The model under review builds one solid part; all positions refer to its coordinate system, in mm. Face numbers are marked on the shaded views. A direction names the side the tool comes from. Round coordinates to 2 decimals unless told otherwise and drop trailing zeros. Loops run counter-clockwise (first coordinate to the right, second up) from the corner with the lowest first, then second, coordinate; pieces in that order, holes last. Notation, with made-up numbers: M -20,46 L 24,46 A9 ccw 24,53 Z; hole C 0,-20 d9. An arc over 180 degrees is marked long. Return JSON: item names as keys, results as strings. Group by question number.
Q1. Consider section B-B (x = -20.5). State the section outline as (y, z) points.
Q2. Consider section A-A (x = 12.7). Count the separate pieces of the cut face and the enclosed holes in it, and give its area (3 significant figures).
Q3. For the marked faces 4, 5, 6, 7 and 8, list the 3-axis set-ups (+Z, -Z, +X, -X, +Y, -Y) from which the entire face can be reached by the end or side of a thin tool; tool diameter is ignored.
Q4. To check wall thickness, follow line 1 along X through (y, z) = (12.7, 4.9); line 2 along Z through (x, y) = (-18.5, 32.5); line 3 along X through (y, z) = (32.5, -5.25). State the ranges of each line that lie inside material, in increasing order.
Q5. Draft analysis for pull direction X (two halves, no side actions). For the marked faces 1, 2 and 3, state which applies: pulls with the +X half, pulls with the -X half, needs draft (parallel to the pull), parting line crosses it, or undercut.
Q6. Clearance check with flat-ended pins moving along their axes: pin 1 Ø6 at (x, z) = (11, 4.5) entering from +Y; pin 2 Ø3.5 at (y, z) = (33.5, -2) entering from +X; pin 3 Ø3.5 at (y, z) = (16, 0) entering from -X; pin 4 Ø6 at (x, z) = (18, -3) entering from +Y. State where each tip first meets the part, or that it passes through.
from build123d import *

# Parameters (mm, degrees)
SKETCH1_W                = 38.1
SKETCH1_H                = 12.7
SKETCH1_R                = 4.05
BOSS_EXTRUDE1_DEPTH      = 25.4
SKETCH5_R                = 1.7526
CUT_EXTRUDE2_DEPTH       = 35.195796525
SKETCH6_W                = 49.584
SKETCH6_H                = 12.7
BOSS_EXTRUDE4_DEPTH      = 19.05
CUT_EXTRUDE3_DEPTH       = 67.893183937
CUT_EXTRUDE4_DEPTH       = 67.893183937
CUT_EXTRUDE5_DEPTH       = 53.194652565
CHAMFER1_SIZE            = 0.6
SKETCH10_W               = 12.7
SKETCH10_H               = 25.4
CUT_EXTRUDE6_DEPTH       = 53.194652565
CHAMFER2_SIZE            = 0.6
CHAMFER3_SIZE            = 0.3
BOSS_EXTRUDE5_DEPTH      = 1.5875
BOSS_EXTRUDE5_DEPTH_BACK = 1.5875
SKETCH14_R               = 4.7625
BOSS_EXTRUDE6_DEPTH      = 2.54
SKETCH15_R               = 1.7526
CUT_EXTRUDE7_DEPTH       = 53.870117777
CHAMFER4_SIZE            = 0.4
SKETCH18_R               = 4.1
BOSS_EXTRUDE7_DEPTH      = 6.35


with BuildPart() as part:
    # Sketch1 → Boss-Extrude1 (new body)
    with BuildSketch(Plane(origin=(0, 0, 0), x_dir=(1, 0, 0), z_dir=(0, 1, 0))):
        Rectangle(SKETCH1_W, SKETCH1_H)
        with Locations(Location((12.7, 0, 0), (0, 0, 270))):
            Circle(SKETCH1_R, mode=Mode.SUBTRACT)
        with Locations(Location((-12.7, 0, 0), (0, 0, 90))):
            Circle(SKETCH1_R, mode=Mode.SUBTRACT)
    extrude(amount=BOSS_EXTRUDE1_DEPTH)

    # Sketch5 → Cut-Extrude2 (cut, through all)
    with BuildSketch(Plane.XY.offset(6.35)):
        with Locations((12.7, 12.7)):
            Circle(SKETCH5_R)
        with Locations((-12.7, 12.7)):
            Circle(SKETCH5_R)
    extrude(amount=-CUT_EXTRUDE2_DEPTH, mode=Mode.SUBTRACT)

    # Sketch6 → Boss-Extrude4 (add)
    with BuildSketch(Plane(origin=(0, 25.4, 0), x_dir=(1, 0, 0), z_dir=(0, 1, 0))):
        Rectangle(SKETCH6_W, SKETCH6_H)
    extrude(amount=BOSS_EXTRUDE4_DEPTH)

    # Sketch7 → Cut-Extrude3 (cut, through all)
    with BuildSketch(Plane.ZY.offset(24.792)):
        Polygon((0, 40.6552014), (-4.962499981, 37.7901007), (-4.962499981, 32.0598993), (0, 29.1947986), (4.962499981, 32.0598993), (4.962499981, 37.7901007), align=None)
    extrude(amount=-CUT_EXTRUDE3_DEPTH, mode=Mode.SUBTRACT)

    # Sketch8 → Cut-Extrude4 (cut, through all)
    with BuildSketch(Plane.ZY.offset(24.792)):
        with BuildLine():
            Line((-6.35, 37.7901007), (-6.35, 44.45))
            Line((-6.35, 44.45), (6.35, 44.45))
            Line((6.35, 44.45), (6.35, 37.7901007))
            ThreePointArc((6.35, 37.7901007), (0, 44.1401007), (-6.35, 37.7901007))
        make_face()
    extrude(amount=-CUT_EXTRUDE4_DEPTH, mode=Mode.SUBTRACT)

    # Sketch9 → Cut-Extrude5 (cut, through all)
    with BuildSketch(Plane(origin=(0, 0, -6.35), x_dir=(-1, 0, 0), z_dir=(0, 0, -1))):
        Polygon((19.05, 25.4), (24.792, 26.9875), (24.792, 25.4), align=None)
        Polygon((-24.792, 25.4), (-19.05, 25.4), (-24.792, 26.9875), align=None)
    extrude(amount=-CUT_EXTRUDE5_DEPTH, mode=Mode.SUBTRACT)

    # Chamfer1
    chamfer1_edges = [part.edges().sort_by_distance(p)[0] for p in [
        (19.05, 0, 0),
        (24.792, 32.38880035, 6.35),
        (24.792, 44.1401007, 0),
        (24.792, 32.38880035, -6.35),
        (21.921, 26.19375, -6.35),
        (19.05, 12.7, -6.35),
        (19.05, 12.7, 6.35),
        (-21.921, 26.19375, 6.35),
        (-24.792, 32.38880035, 6.35),
        (-24.792, 44.1401007, 0),
        (-24.792, 32.38880035, -6.35),
        (-21.921, 26.19375, -6.35),
        (0, 0, 6.35),
        (0, 0, -6.35),
        (-19.05, 12.7, 6.35),
        (-19.05, 0, 0),
        (-19.05, 12.7, -6.35),
    ]]
    chamfer(chamfer1_edges, length=CHAMFER1_SIZE)

    # Sketch10 → Cut-Extrude6 (cut, through all)
    with BuildSketch(Plane.XY.offset(6.35)):
        with Locations((0, 35.525)):
            Rectangle(SKETCH10_W, SKETCH10_H)
    extrude(amount=-CUT_EXTRUDE6_DEPTH, mode=Mode.SUBTRACT)

    # Chamfer2
    chamfer2_edges = [part.edges().sort_by_distance(p)[0] for p in [
        (-6.35, 44.1401007, 0),
        (6.35, 44.1401007, 0),
        (6.35, 30.30755035, -6.35),
        (-6.35, 30.30755035, -6.35),
        (-6.35, 22.825, 0),
        (6.35, 30.30755035, 6.35),
        (-6.35, 30.30755035, 6.35),
        (0, 22.825, 6.35),
        (0, 22.825, -6.35),
        (6.35, 22.825, 0),
    ]]
    chamfer(chamfer2_edges, length=CHAMFER2_SIZE)

    # Chamfer3
    chamfer3_edges = [part.edges().sort_by_distance(p)[0] for p in [
        (6.35, 34.925, 4.962499981),
        (6.35, 39.22265105, 2.481249991),
        (6.35, 39.22265105, -2.48124999),
        (6.35, 34.925, -4.962499981),
        (6.35, 30.62734895, -2.48124999),
        (6.35, 30.62734895, 2.481249991),
        (-6.35, 39.22265105, -2.48124999),
        (-6.35, 39.22265105, 2.481249991),
        (-6.35, 34.925, 4.962499981),
        (-6.35, 30.62734895, 2.481249991),
        (-6.35, 30.62734895, -2.48124999),
        (-6.35, 34.925, -4.962499981),
        (24.792, 39.22265105, 2.481249991),
        (24.792, 34.925, 4.962499981),
        (24.792, 30.62734895, 2.481249991),
        (24.792, 30.62734895, -2.48124999),
        (24.792, 34.925, -4.962499981),
        (24.792, 39.22265105, -2.481249991),
        (-24.792, 39.22265105, 2.481249991),
        (-24.792, 39.22265105, -2.48124999),
        (-24.792, 34.925, -4.962499981),
        (-24.792, 30.62734895, -2.48124999),
        (-24.792, 30.62734895, 2.481249991),
        (-24.792, 34.925, 4.962499981),
    ]]
    chamfer(chamfer3_edges, length=CHAMFER3_SIZE)

    # Sketch13 → Boss-Extrude5 (add, two sides: drawn at the far end of the back side and taken through both)
    with BuildSketch(Plane(origin=(0, 0, 0), x_dir=(0, -1, 0), z_dir=(0, 0, -1)).offset(-BOSS_EXTRUDE5_DEPTH_BACK)):
        Polygon((-25.4, 19.05), (-26.9875, 24.792), (-13, 19.05), align=None)
        Polygon((-26.9875, -24.792), (-13, -19.05), (-25.4, -19.05), align=None)
    extrude(amount=BOSS_EXTRUDE5_DEPTH + BOSS_EXTRUDE5_DEPTH_BACK)

    # Sketch14 → Boss-Extrude6 (add)
    with BuildSketch(Plane(origin=(0, 0, -6.35), x_dir=(-1, 0, 0), z_dir=(0, 0, -1))):
        with Locations(Location((-12.7, 12.7, 0), (0, 0, 180))):
            Circle(SKETCH14_R)
        with Locations(Location((12.7, 12.7, 0), (0, 0, 180))):
            Circle(SKETCH14_R)
    extrude(amount=BOSS_EXTRUDE6_DEPTH)

    # Sketch15 → Cut-Extrude7 (cut, through all)
    with BuildSketch(Plane.XY.offset(6.35)):
        with Locations((12.7, 12.7)):
            Circle(SKETCH15_R)
        with Locations((-12.7, 12.7)):
            Circle(SKETCH15_R)
    extrude(amount=-CUT_EXTRUDE7_DEPTH, mode=Mode.SUBTRACT)

    # Chamfer4
    chamfer4_edges = [part.edges().sort_by_distance(p)[0] for p in [
        (7.9375, 12.7, -6.35),
        (7.9375, 12.7, -8.89),
        (-17.4625, 12.7, -6.35),
        (-17.4625, 12.7, -8.89),
        (10.9474, 12.7, -8.89),
        (-14.4526, 12.7, -8.89),
    ]]
    chamfer(chamfer4_edges, length=CHAMFER4_SIZE)

    # Sketch18 → Boss-Extrude7 (add)
    with BuildSketch(Plane.XZ.offset(-25.4)):
        with Locations((-12.7, 0)):
            Circle(SKETCH18_R)
        with Locations((12.7, 0)):
            Circle(SKETCH18_R)
    extrude(amount=BOSS_EXTRUDE7_DEPTH)


solid = part.part
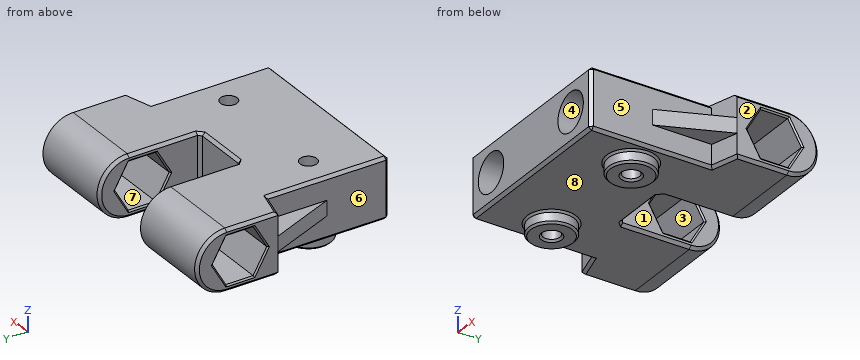
Values:
{
 "1": {"outline": "M 16.53,-1.59 L 25.8,-1.59 L 25.8,-5.75 L 26.42,-6.35 L 37.79,-6.35 A6.35 ccw 37.79,6.35 L 26.42,6.35 L 25.8,5.75 L 25.8,1.59 L 16.53,1.59 Z; hole M 29.19,0 L 32.06,-4.96 L 37.79,-4.96 L 40.66,0 L 37.79,4.96 L 32.06,4.96 Z"},
 "2": {"separate pieces": "3", "enclosed holes": "1", "area": "302 mm2"},
 "3": {"face 4": "-Y", "face 5": "+X, -Y", "face 6": "-X, -Y", "face 7": "+X, -X", "face 8": "-Z"},
 "4": {"line 1": "x = -19.05 to -14.45, -10.95 to 10.95, 14.45 to 19.05", "line 2": "z = -6.35 to -4.96, 4.96 to 6.35", "line 3": "x = -24.78 to -6.36, 6.36 to 24.78"},
 "5": {"face 1": "undercut", "face 2": "pulls with the +X half", "face 3": "needs draft"},
 "6": {"pin 1": "stops at y = 43.96", "pin 2": "passes through", "pin 3": "stops at x = -21", "pin 4": "stops at y = 44.14"}
}
